```python
from build123d import *

# Parameters (mm, degrees)
BOSS_EXTRUDE1_DEPTH                     = 35
SKETCH2_W                               = 96
SKETCH2_H                               = 28
CUT_EXTRUDE1_DEPTH                      = 2.5
SKETCH3_W                               = 42
SKETCH3_H                               = 19
CUT_EXTRUDE2_DEPTH                      = 56
SKETCH4_R                               = 2
CUT_EXTRUDE3_DEPTH                      = 6
CUT_EXTRUDE4_START                      = -18
SKETCH5_W                               = 65
SKETCH5_H                               = 22
CUT_EXTRUDE4_DEPTH                      = 21
CHAMFER2_SIZE                           = 20
BOSS_EXTRUDE4_DEPTH                     = 15
CUT_EXTRUDE5_REACH                      = 344.352
SKETCH10_R                              = 2.3
MOTOR_DRIVER_PATTERNED_COUNT            = 3
CHAMFER2_OF_MOTOR_DRIVER_PATTERNED_SIZE = 20
CUT_EXTRUDE6_DEPTH                      = 25
CUT_EXTRUDE6_DRAFT                      = -26.75
SKETCH11_R                              = 3.15
SKETCH11_R_2                            = 1.65
RASPBERRYPI5_STANDOFF_DEPTH             = 5
SKETCH13_R                              = 3.15
SKETCH13_R_2                            = 1.65
BOSS_EXTRUDE6_DEPTH                     = 5


with BuildPart() as part:
    # Sketch1 → Boss-Extrude1 (new body)
    with BuildSketch(Plane(origin=(0, 0, 0), x_dir=(1, 0, 0), z_dir=(0, 1, 0))):
        Polygon((-20, 144.337567297), (100, 144.337567297), (135, -54.848275573), (75, -158.771324027), (-115, -89.489291724), (-175, 14.43375673), align=None)
    extrude(amount=BOSS_EXTRUDE1_DEPTH)

    # Sketch2 → Cut-Extrude1 (cut)
    with BuildSketch(Plane(origin=(0, 0, -144.337567297), x_dir=(-1, 0, 0), z_dir=(0, 0, -1))):
        with Locations((-40, 14)):
            Rectangle(SKETCH2_W, SKETCH2_H)
    cut_extrude1 = extrude(amount=-CUT_EXTRUDE1_DEPTH, mode=Mode.SUBTRACT)

    # Sketch3 → Cut-Extrude2 (cut)
    with BuildSketch(Plane(origin=(0, 0, -141.837567297), x_dir=(-1, 0, 0), z_dir=(0, 0, -1))):
        with Locations((-61, 18.5)):
            Rectangle(SKETCH3_W, SKETCH3_H)
        with Locations((-19, 18.5)):
            Rectangle(SKETCH3_W, SKETCH3_H)
        Polygon((-88, 9), (-88, 0), (8, 0), (8, 9), (2, 9), (-40, 9), (-82, 9), align=None)
    cut_extrude2 = extrude(amount=-CUT_EXTRUDE2_DEPTH, mode=Mode.SUBTRACT)

    # Sketch4 → Cut-Extrude3 (cut)
    with BuildSketch(Plane(origin=(0, 0, -141.837567297), x_dir=(-1, 0, 0), z_dir=(0, 0, -1))):
        with Locations((-85, 16.25)):
            Circle(SKETCH4_R)
        with Locations((5, 16.25)):
            Circle(SKETCH4_R)
    cut_extrude3 = extrude(amount=-CUT_EXTRUDE3_DEPTH, mode=Mode.SUBTRACT)

    # Sketch5 → Cut-Extrude4 (cut)
    with BuildSketch(Plane(origin=(0, 0, -85.837567297), x_dir=(-1, 0, 0), z_dir=(0, 0, -1)).offset(CUT_EXTRUDE4_START)):
        with Locations((-40, 25.5)):
            Rectangle(SKETCH5_W, SKETCH5_H)
    cut_extrude4 = extrude(amount=CUT_EXTRUDE4_DEPTH, mode=Mode.SUBTRACT)

    # Chamfer2
    chamfer2_edges = [part.edges().sort_by_distance(p)[0] for p in [
        (40, 35, -67.837567297),
    ]]
    chamfer(chamfer2_edges, length=CHAMFER2_SIZE)

    # Sketch7 → Boss-Extrude4 (add)
    with BuildSketch(Plane(origin=(36, 0, 0), x_dir=(0, 0, -1), z_dir=(1, 0, 0))):
        with BuildLine():
            Line((95.437567297, 72.3), (95.437567297, 35))
            Line((95.437567297, 35), (137.737567297, 35))
            Line((137.737567297, 35), (137.737567297, 72.3))
            Line((137.737567297, 72.3), (132.737567297, 77.3))
            Line((132.737567297, 77.3), (122.837567297, 77.3))
            Line((122.837567297, 77.3), (122.837567297, 85.3))
            Line((122.837567297, 85.3), (117.837567297, 85.3))
            Line((117.837567297, 85.3), (117.837567297, 74.106544768))
            ThreePointArc((117.837567297, 74.106544768), (116.587567297, 38.15), (115.337567297, 74.106544768))
            Line((115.337567297, 74.106544768), (115.337567297, 85.3))
            Line((115.337567297, 85.3), (110.337567297, 85.3))
            Line((110.337567297, 85.3), (110.337567297, 77.3))
            Line((110.337567297, 77.3), (100.437567297, 77.3))
            Line((100.437567297, 77.3), (95.437567297, 72.3))
        make_face()
    boss_extrude4 = extrude(amount=-BOSS_EXTRUDE4_DEPTH)

    # Cut-Extrude5: up to this face of the body (flat: up to its plane)
    cut_extrude5_end = Plane(part.part.faces().sort_by_distance((28.5, 81.3, -110.337567297))[0])
    # Sketch10 → Cut-Extrude5 (cut, up to the picked face)
    with BuildSketch(Plane(origin=(0, 0, -122.837567297), x_dir=(-1, 0, 0), z_dir=(0, 0, -1)), mode=Mode.PRIVATE) as cut_extrude5_sk1:
        with Locations(Location((-28.5, 81.3, 0), (0, 0, 90))):
            Circle(SKETCH10_R)
    cut_extrude5_tool1 = split(extrude(cut_extrude5_sk1.sketch, amount=-CUT_EXTRUDE5_REACH, mode=Mode.PRIVATE), bisect_by=cut_extrude5_end, keep=Keep.BOTH, mode=Mode.PRIVATE)
    cut_extrude5 = cut_extrude5_tool1.solids().sort_by(Axis((28.5, 81.3, -122.837567), (0, 0, 1)))[0]
    add(cut_extrude5, mode=Mode.SUBTRACT)

    # Motor/Driver Patterned: Cut-Extrude1, Cut-Extrude2, Cut-Extrude3, Cut-Extrude4, Boss-Extrude4, Cut-Extrude5 ×3 about axis
    motor_driver_patterned_axis = Axis((0, 0, 0), (0, 1, 0))
    add([cut_extrude1.rotate(motor_driver_patterned_axis, i * 360 / MOTOR_DRIVER_PATTERNED_COUNT) for i in range(1, MOTOR_DRIVER_PATTERNED_COUNT)], mode=Mode.SUBTRACT)
    add([cut_extrude2.rotate(motor_driver_patterned_axis, i * 360 / MOTOR_DRIVER_PATTERNED_COUNT) for i in range(1, MOTOR_DRIVER_PATTERNED_COUNT)], mode=Mode.SUBTRACT)
    add([cut_extrude3.rotate(motor_driver_patterned_axis, i * 360 / MOTOR_DRIVER_PATTERNED_COUNT) for i in range(1, MOTOR_DRIVER_PATTERNED_COUNT)], mode=Mode.SUBTRACT)
    add([cut_extrude4.rotate(motor_driver_patterned_axis, i * 360 / MOTOR_DRIVER_PATTERNED_COUNT) for i in range(1, MOTOR_DRIVER_PATTERNED_COUNT)], mode=Mode.SUBTRACT)
    add([boss_extrude4.rotate(motor_driver_patterned_axis, i * 360 / MOTOR_DRIVER_PATTERNED_COUNT) for i in range(1, MOTOR_DRIVER_PATTERNED_COUNT)])
    add([cut_extrude5.rotate(motor_driver_patterned_axis, i * 360 / MOTOR_DRIVER_PATTERNED_COUNT) for i in range(1, MOTOR_DRIVER_PATTERNED_COUNT)], mode=Mode.SUBTRACT)

    # Chamfer2 of Motor/Driver Patterned
    chamfer2_of_motor_driver_patterned_edges = [part.edges().sort_by_distance(p)[0] for p in [
        (-78.74905661, 35, -0.722232503),
        (38.74905661, 35, 68.5597998),
    ]]
    chamfer(chamfer2_of_motor_driver_patterned_edges, length=CHAMFER2_OF_MOTOR_DRIVER_PATTERNED_SIZE)


with BuildPart() as cut_extrude6_tool:
    # Sketch16 → Cut-Extrude6 (with draft: the straight prism first)
    with BuildSketch(Plane(origin=(0, 10, 0), x_dir=(1, 0, 0), z_dir=(0, 1, 0))):
        Polygon((4.64219366, 24.61990329), (-21.829310641, 12.295153393), (-9.504560743, -14.176350908), (16.966943558, -1.851601011), align=None)
    extrude(amount=CUT_EXTRUDE6_DEPTH)
    # Cut-Extrude6: the draft: its side faces are tilted about the plane it starts from
    cut_extrude6_sides = [cut_extrude6_tool.faces().sort_by_distance(p)[0] for p in [
        (-8.59355849, 22.5, -18.457528341),
        (-15.666935692, 22.5, 0.940598758),
        (3.731191407, 22.5, 8.01397596),
        (10.804568609, 22.5, -11.38415114),
    ]]
    draft(cut_extrude6_sides, Plane(origin=(0, 10, 0), x_dir=(1, 0, 0), z_dir=(0, 1, 0)), CUT_EXTRUDE6_DRAFT)


with BuildPart() as part_1:
    add(part.part)

    # Cut-Extrude6: cut by cut_extrude6_tool
    add(cut_extrude6_tool.part, mode=Mode.SUBTRACT)

    # Sketch11 → RaspberryPi5 Standoff (add)
    # profile 1 of 4: a face of its own
    with BuildSketch(Plane(origin=(0, 35, 0), x_dir=(1, 0, 0), z_dir=(0, 1, 0))):
        with Locations(Location((-10.300566951, 37.647855731, 0), (0, 0, 270))):
            Circle(SKETCH11_R)
        with Locations(Location((-10.300566951, 37.647855731, 0), (0, 0, 270))):
            Circle(SKETCH11_R_2, mode=Mode.SUBTRACT)
    # profile 2 of 4: a face of its own
    with BuildSketch(Plane(origin=(0, 35, 0), x_dir=(1, 0, 0), z_dir=(0, 1, 0))):
        with Locations(Location((-47.555881138, 82.100544792, 0), (0, 0, 270))):
            Circle(SKETCH11_R)
        with Locations(Location((-47.555881138, 82.100544792, 0), (0, 0, 270))):
            Circle(SKETCH11_R_2, mode=Mode.SUBTRACT)
    # profile 3 of 4: a face of its own
    with BuildSketch(Plane(origin=(0, 35, 0), x_dir=(1, 0, 0), z_dir=(0, 1, 0))):
        with Locations(Location((-85.110739139, 50.626227634, 0), (0, 0, 270))):
            Circle(SKETCH11_R)
        with Locations(Location((-85.110739139, 50.626227634, 0), (0, 0, 270))):
            Circle(SKETCH11_R_2, mode=Mode.SUBTRACT)
    # profile 4 of 4: a face of its own
    with BuildSketch(Plane(origin=(0, 35, 0), x_dir=(1, 0, 0), z_dir=(0, 1, 0))):
        with Locations(Location((-47.855424951, 6.173538573, 0), (0, 0, 270))):
            Circle(SKETCH11_R)
        with Locations(Location((-47.855424951, 6.173538573, 0), (0, 0, 270))):
            Circle(SKETCH11_R_2, mode=Mode.SUBTRACT)
    extrude(amount=RASPBERRYPI5_STANDOFF_DEPTH)

    # Sketch13 → Boss-Extrude6 (add)
    # profile 1 of 4: a face of its own
    with BuildSketch(Plane(origin=(0, 10, 0), x_dir=(1, 0, 0), z_dir=(0, 1, 0))):
        with Locations(Location((7.566649181, 8.861795539, 0), (0, 0, 270))):
            Circle(SKETCH13_R)
        with Locations(Location((7.566649181, 8.861795539, 0), (0, 0, 270))):
            Circle(SKETCH13_R_2, mode=Mode.SUBTRACT)
    # profile 2 of 4: a face of its own
    with BuildSketch(Plane(origin=(0, 10, 0), x_dir=(1, 0, 0), z_dir=(0, 1, 0))):
        with Locations(Location((-11.652388188, -0.086310551, 0), (0, 0, 270))):
            Circle(SKETCH13_R)
        with Locations(Location((-11.652388188, -0.086310551, 0), (0, 0, 270))):
            Circle(SKETCH13_R_2, mode=Mode.SUBTRACT)
    # profile 3 of 4: a face of its own
    with BuildSketch(Plane(origin=(0, 10, 0), x_dir=(1, 0, 0), z_dir=(0, 1, 0))):
        with Locations(Location((-7.566649181, -8.861795539, 0), (0, 0, 270))):
            Circle(SKETCH13_R)
        with Locations(Location((-7.566649181, -8.861795539, 0), (0, 0, 270))):
            Circle(SKETCH13_R_2, mode=Mode.SUBTRACT)
    # profile 4 of 4: a face of its own
    with BuildSketch(Plane(origin=(0, 10, 0), x_dir=(1, 0, 0), z_dir=(0, 1, 0))):
        with Locations(Location((11.652388188, 0.086310551, 0), (0, 0, 270))):
            Circle(SKETCH13_R)
        with Locations(Location((11.652388188, 0.086310551, 0), (0, 0, 270))):
            Circle(SKETCH13_R_2, mode=Mode.SUBTRACT)
    extrude(amount=BOSS_EXTRUDE6_DEPTH)


solid = part_1.part
```
Geometry check sheet. Reference: the model listing, model coordinates, mm. A direction names the side the tool comes from. Coordinates: 2 decimals unless noted, no trailing zeros. Write each loop counter-clockwise with the first axis right and the second up, starting at its lowest first coordinate (ties: lowest second). Pieces come first, ordered by that corner, then holes. Notation, with made-up numbers: M 68.25,64 L 103.25,64 A31 cw 103.25,96 Z; hole C 38.25,40 d3. An arc over 180 degrees is marked long. One line per item, written item: value. Start each with the question number.
(1) Sectioned sample at A-A, the plane y = 58.5. Enter the section's corners in (x, z).
(2) Tool access check on faces 4 (the face through (-69.983, 24.86, -5.258)), 5 (the face through (40, 14.5, -77)), 6 (the face through (82.07, 71.68, 71.63)). Record the directions out of +Z, -Z, +X, -X, +Y, -Y that give a thin tool (end or side, any length) a straight path to the whole face; none if there is none.
(3) Depth check by flat-ended pin: pin 1 (3 mm diameter, centred on x = -13, z = -1, fed in from +Y); pin 2 (1 mm diameter, centred on x = -7, z = 61, fed in from +Y); pin 3 (9 mm diameter, centred on x = 27, y = 81, fed in from -Z). Enter the tip coordinate at first touch or a pass-through.
(4) Scan lines: line 1 along Z through (x, y) = (22.5, 23); line 2 along X through (y, z) = (16, -140); line 3 along X through (y, z) = (81.3, -113.65). Record each from-to range of solid material in increasing order. Write a range as [from, to].
(5) Release check for a two-part mould opening along X. For faces 1 (the face through (36, 72, -126)), 2 (the face through (-78.98, 14.75, -1.12)), 3 (the face through (-96, 9, 61)) record: released by +X, released by -X, zero draft, split by the parting line, or undercut.
Filled sheet:
1. outline: M -137.28,37.69 L -134.42,36.04 L -126.92,49.03 L -129.78,50.68 Z; M -103.51,18.19 L -100.65,16.54 L -93.15,29.53 L -96.01,31.18 Z; M 21,-137.74 L 36,-137.74 L 36,-134.43 L 21,-134.43 Z; M 21,-98.74 L 36,-98.74 L 36,-95.44 L 21,-95.44 Z; M 64.65,78.9 L 72.15,65.91 L 75.01,67.56 L 67.51,80.55 Z; M 98.42,98.39 L 105.92,85.4 L 108.78,87.06 L 101.28,100.05 Z
2. face 4: +Y
2. face 5: -Z, +Y
2. face 6: -Z, +X, +Y
3. pin 1: y = 15
3. pin 2: y = 35
3. pin 3: z = -133.54
4. line 1: [-59.84, -1.79], [6.5, 80.7], [96.71, 139.63]
4. line 2: [-25.18, -6.98], [-3.02, -2], [82, 83.02], [86.98, 100.76]
4. line 3: [21, 26.2], [30.8, 36]
5. face 1: released by +X
5. face 2: undercut
5. face 3: zero draft
